Geometry check sheet. Reference: the model listing, model coordinates, mm. Coordinates: 2 decimals unless noted, no trailing zeros. Write each loop counter-clockwise with the first axis right and the second up, starting at its lowest first coordinate (ties: lowest second). Pieces come first, ordered by that corner, then holes. Notation, with made-up numbers: (19, -33.75) -> (71, -33.75) arc R29 ccw to (71, -3.75) -> close; hole circle Ø7 at (83.5, 52). An arc over 180 degrees is marked (long way). Answer in a Markdown table with one row per item. Add a question column.
1. Cross-section at A-A on y = 55. Record the cut outline in (x, z).
2. Cross-section at D-D on y = 13.75. Record the cut outline in (x, z).
3. Depth check by flat-ended pin: P1, Ø4, axis at x = -11.75, y = -56.75, coming from the -Z side. Enter the tip coordinate at first touch or a pass-through.
4. Cross-section at C-C on x = 25.5. Record the cut outline in (y, z), and give its area (3 significant figures).
5. Scan lines: L1, parallel to Y at x = 25.5, z = 1.65; L2, parallel to Y at x = 11, z = 1.55; L3, parallel to Y at x = 27, z = 0.4. Record each from-to range of solid material in increasing order. Write a range as from..to.
6. Cross-section at B-B on x = 11.25. Record the cut outline in (y, z), and give its area (3 significant figures).
7. Mould release check, pull along X, two halves, no side actions. Record for faces 1 (the flat face through (16, -20, 2)), 2 (the cylindrical face through (-11.952, -29.037, 0.986)): pulls with the +X half, pulls with the -X half, needs draft (parallel to the pull), parting line crosses it, or undercut.
Autodesk Inventor part; units mm, degrees
ref_plane "YZ Plane" through (0, 0, 0) normal (1, 0, 0) x (0, 1, 0)
ref_plane "XZ Plane" through (0, 0, 0) normal (0, 1, 0) x (-1, 0, 0)
ref_plane "XY Plane" through (0, 0, 0) normal (0, 0, 1) x (1, 0, 0)
sketch "スケッチ1" plane through (0, 0, 0) normal (0, 0, 1) x (1, 0, 0)
  circle A0 centre (-4.75, 48) radius 1.2
  circle A1 centre (4.75, 48) radius 1.2
  circle A2 centre (-4.75, -48) radius 1.2
  circle A3 centre (4.75, -48) radius 1.2
  line L0 (-4.75, -48) -> (4.75, -48) construction
  line L1 (4.75, -48) -> (4.75, 48) construction
  line L2 (4.75, 48) -> (-4.75, 48) construction
  line L3 (-4.75, 48) -> (-4.75, -48) construction
  line L4 (-4.75, -48) -> (4.75, 48) construction
  line L5 (4.75, -48) -> (-4.75, 48) construction
  line L6 (-17.75, 61) -> (50.25, 61)
  line L7 (50.25, 61) -> (50.25, -104)
  line L8 (50.25, -104) -> (-17.75, -104)
  line L9 (-17.75, -104) -> (-17.75, 61)
  circle A4 centre (44.25, 55) radius 1.55
  line L10 (16.25, 61) -> (16.25, -104) construction
  line L11 (16.25, -21.5) -> (50.25, -21.5) construction
  circle A5 centre (21.25, 55) radius 1.55
  circle A6 centre (33.25, 55) radius 1.55
  line L12 (16.25, 19.75) -> (50.25, 19.75) construction
  line L13 (16.25, 40.375) -> (50.25, 40.375) construction
  circle A7 centre (44.25, 25.75) radius 1.55
  circle A8 centre (44.25, -15.5) radius 1.55
  circle A9 centre (44.25, 13.75) radius 1.55
  circle A10 centre (44.25, -98) radius 1.55
  circle A11 centre (21.25, -98) radius 1.55
  circle A12 centre (33.25, -98) radius 1.55
  circle A13 centre (44.25, -68.75) radius 1.55
  circle A14 centre (44.25, -27.5) radius 1.55
  circle A15 centre (44.25, -56.75) radius 1.55
  circle A16 centre (-11.75, 55) radius 1.55
  circle A17 centre (11.25, 55) radius 1.55
  circle A18 centre (-0.75, 55) radius 1.55
  circle A19 centre (-11.75, 25.75) radius 1.55
  circle A20 centre (-11.75, -15.5) radius 1.55
  circle A21 centre (-11.75, 13.75) radius 1.55
  circle A22 centre (-11.75, -27.5) radius 1.55
  circle A23 centre (-11.75, -56.75) radius 1.55
  circle A24 centre (11.25, -98) radius 1.55
  circle A25 centre (-0.75, -98) radius 1.55
  circle A26 centre (-11.75, -98) radius 1.55
  circle A27 centre (-11.75, -68.75) radius 1.55
  circle A28 centre (-4.75, 38) radius 1.2
  circle A29 centre (4.75, 38) radius 1.2
  circle A30 centre (-4.75, -58) radius 1.2
  circle A31 centre (4.75, -58) radius 1.2
  circle A32 centre (-4.75, 28) radius 1.2
  circle A33 centre (4.75, 28) radius 1.2
  circle A34 centre (-4.75, -68) radius 1.2
  circle A35 centre (4.75, -68) radius 1.2
  circle A36 centre (-4.75, 18) radius 1.2
  circle A37 centre (4.75, 18) radius 1.2
  circle A38 centre (-4.75, -78) radius 1.2
  circle A39 centre (4.75, -78) radius 1.2
  circle A40 centre (-4.75, 8) radius 1.2
  circle A41 centre (4.75, 8) radius 1.2
  circle A42 centre (-4.75, -88) radius 1.2
  circle A43 centre (4.75, -88) radius 1.2
  circle A44 centre (25.5, 36.25) radius 10.75
  line L14 (14.75, 47) -> (36.25, 47) construction
  line L15 (36.25, 47) -> (36.25, -90) construction
  line L16 (36.25, -90) -> (14.75, -90) construction
  line L17 (14.75, -90) -> (14.75, 47) construction
  circle A45 centre (25.5, -0.75) radius 10.75
  circle A46 centre (25.5, -37.75) radius 10.75
  circle A47 centre (25.5, -74.75) radius 10.75
  circle A48 centre (4.75, 48) radius 2.75 construction
  point P0 (0, 0)
  dimension "d0" = 2.4
  dimension "d1" = 9.5
  dimension "d2" = 96
  dimension "d3" = 13
  dimension "d4" = 13
  dimension "d7" = 165
  dimension "d8" = 68
  dimension "d16" = 3.1
  dimension "d17" = 6
  dimension "d18" = 6
  dimension "d19" = 5
  dimension "d20" = 17
  dimension "d21" = 41.25
  dimension "d22" = 20.625
  dimension "d25" = 10
  dimension "d30" = 10
  dimension "d31" = 8
  dimension "d32" = 8
  dimension "d35" = 37
  dimension "d40" = 8
  dimension "d41" = 5.5
extrude "押し出し1" add sketch "スケッチ1" along normal blind 2
equation "\"d1\" = d20_1"
equation "\"d4\" = d3"
equation "\"d8\" = 足_短辺"
equation "\"d18\" = d17"
equation "\"d20\" = 0.25 * d8"
equation "\"d21\" = 0.25 * d7"
equation "\"d22\" = 0.5 * d21"
equation "\"d31\" = d32"
equation "\"d40\" = d31"
equation "\"H_head\" = 28.5"
equation "\"H_leg\" = 306"
equation "\"足の面積\" = 12720.125"
equation "\"現在の面積\" = 11560"
equation "\"足_短辺\" = 68"
equation "\"円柱\" = 313.5"
equation "\"胴体中心から手先\" = 342"
equation "\"H_leg_1\" = 186.2"
equation "\"H_leg_MAX\" = 399"
equation "\"H_head_1\" = 26.6"
equation "\"H_head_MAX\" = 142.5"
properties part number "足裏_メインフレーム_1_3" material "GFRP"
Results found:
| question | item | result |
|---|---|---|
| 1 | outline | (-17.75, 0) -> (-13.3, 0) -> (-13.3, 2) -> (-17.75, 2) -> close; (-10.2, 0) -> (-2.3, 0) -> (-2.3, 2) -> (-10.2, 2) -> close; (0.8, 0) -> (9.7, 0) -> (9.7, 2) -> (0.8, 2) -> close; (12.8, 0) -> (19.7, 0) -> (19.7, 2) -> (12.8, 2) -> close; (22.8, 0) -> (31.7, 0) -> (31.7, 2) -> (22.8, 2) -> close; (34.8, 0) -> (42.7, 0) -> (42.7, 2) -> (34.8, 2) -> close; (45.8, 0) -> (50.25, 0) -> (50.25, 2) -> (45.8, 2) -> close |
| 2 | outline | (-17.75, 0) -> (-13.3, 0) -> (-13.3, 2) -> (-17.75, 2) -> close; (-10.2, 0) -> (42.7, 0) -> (42.7, 2) -> (-10.2, 2) -> close; (45.8, 0) -> (50.25, 0) -> (50.25, 2) -> (45.8, 2) -> close |
| 3 | P1 | stops at z = 0 |
| 4 | outline | (-104, 0) -> (-85.5, 0) -> (-85.5, 2) -> (-104, 2) -> close; (-64, 0) -> (-48.5, 0) -> (-48.5, 2) -> (-64, 2) -> close; (-27, 0) -> (-11.5, 0) -> (-11.5, 2) -> (-27, 2) -> close; (10, 0) -> (25.5, 0) -> (25.5, 2) -> (10, 2) -> close; (47, 0) -> (61, 0) -> (61, 2) -> (47, 2) -> close |
| 4 | area | 158 mm^2 |
| 5 | L1 | y = -104..-85.5, -64..-48.5, -27..-11.5, 10..25.5, 47..61 |
| 5 | L2 | y = -104..-99.53, -96.47..53.47, 56.53..61 |
| 5 | L3 | y = -104..-85.39, -64.11..-48.39, -27.11..-11.39, 9.89..25.61, 46.89..61 |
| 6 | outline | (-104, 0) -> (-99.55, 0) -> (-99.55, 2) -> (-104, 2) -> close; (-96.45, 0) -> (53.45, 0) -> (53.45, 2) -> (-96.45, 2) -> close; (56.55, 0) -> (61, 0) -> (61, 2) -> (56.55, 2) -> close |
| 6 | area | 318 mm^2 |
| 7 | face 1 | needs draft |
| 7 | face 2 | undercut |
